Read the model definition and answer for the solid it produces. Units are mm, in the model's axes. Round coordinates to 2 decimals unless told otherwise and drop trailing zeros. Loops run counter-clockwise (first coordinate to the right, second up) from the corner with the lowest first, then second, coordinate; pieces in that order, holes last. Notation, with made-up numbers: (-13.5, 30.5) - (4.5, 30.5) arc R21 cw to (4.5, 45.5) - close; hole circle Ø7 at (62, -37). An arc over 180 degrees is marked (long way). Use CSV: the item, a comma, the result in double quotes. Start each with the question number.
1. Consider line 1 along Y through (x, z) = (0, 1.85); line 2 along Z through (x, y) = (-15, -8.5); line 3 along X through (y, z) = (2, 5.35). Determine where each line is inside the solid, lowest interval first.
2. Find section D-D (x = -11.5). Give the vertices of the cut face in (y, z), and give its area (3 significant figures).
3. Determine the mould class of faces 1 (the cylindrical face through (-0.867, -3.905, 4.479)), 2 (the flat face through (-4.3, 0.3, 3)), 3 (the cylindrical face through (10.2, -0.6, 1.5)) for opening direction X: +X half, -X half, draft (parallel to the pull), parting line (faces both ways), or undercut.
4. Given pin 1 Ø7 at (x, y) = (0, 0) entering from -Z; pin 2 Ø2 at (y, z) = (-9, 2.5) entering from +X; pin 3 Ø2.5 at (x, y) = (0, -11) entering from +Z; pin 4 Ø2 at (y, z) = (-14, 1) entering from +X, each flat-ended and moving along its own axis, determine where each tip first touches the part or whether it passes through.
5. Find section A-A (x = 11). Give the vertices of the cut face in (y, z).
6. Find section B-B (y = 2). Give the vertices of the cut face in (x, z).
7. Find section C-C (z = 4.2). Give the vertices of the cut face in (x, y), and give its area (3 significant figures).
from build123d import *

# Parameters (mm, degrees)
SKETCH1_R           = 18
SKETCH1_R_2         = 1
BOSS_EXTRUDE1_DEPTH = 3
SKETCH2_R           = 4
SKETCH2_R_2         = 3
BOSS_EXTRUDE2_DEPTH = 3
SKETCH3_R           = 3
CUT_EXTRUDE1_DEPTH  = 5


with BuildPart() as part:
    # Sketch1 → Boss-Extrude1 (new body)
    with BuildSketch(Plane.XY):
        Circle(SKETCH1_R)
        with Locations((0, 11)):
            Circle(SKETCH1_R_2, mode=Mode.SUBTRACT)
        with Locations((11, 0)):
            Circle(SKETCH1_R_2, mode=Mode.SUBTRACT)
        with Locations((0, -11)):
            Circle(SKETCH1_R_2, mode=Mode.SUBTRACT)
        with Locations((-11, 0)):
            Circle(SKETCH1_R_2, mode=Mode.SUBTRACT)
    extrude(amount=BOSS_EXTRUDE1_DEPTH)

    # Sketch2 → Boss-Extrude2 (add)
    with BuildSketch(Plane.XY.offset(3)):
        Circle(SKETCH2_R)
        Circle(SKETCH2_R_2, mode=Mode.SUBTRACT)
    extrude(amount=BOSS_EXTRUDE2_DEPTH)

    # Sketch3 → Cut-Extrude1 (cut)
    with BuildSketch(Plane.XY.offset(3)):
        Circle(SKETCH3_R)
    extrude(amount=-CUT_EXTRUDE1_DEPTH, mode=Mode.SUBTRACT)


solid = part.part
Filled sheet:
1,line 1,"y = -18 to -12, -10 to -3, 3 to 10, 12 to 18"
1,line 2,"z = 0 to 3"
1,line 3,"x = -3.46 to -2.24, 2.24 to 3.46"
2,outline,"(-13.85, 0) - (-0.87, 0) - (-0.87, 3) - (-13.85, 3) - close; (0.87, 0) - (13.85, 0) - (13.85, 3) - (0.87, 3) - close"
2,area,"77.9 mm²"
3,face 1,"parting line"
3,face 2,"draft"
3,face 3,"undercut"
4,pin 1,"stops at z = 0"
4,pin 2,"stops at x = 16.12"
4,pin 3,"stops at z = 3"
4,pin 4,"stops at x = 12.45"
5,outline,"(-14.25, 0) - (-1, 0) - (-1, 3) - (-14.25, 3) - close; (1, 0) - (14.25, 0) - (14.25, 3) - (1, 3) - close"
6,outline,"(-17.89, 0) - (-2.24, 0) - (-2.24, 6) - (-3.46, 6) - (-3.46, 3) - (-17.89, 3) - close; (2.24, 0) - (17.89, 0) - (17.89, 3) - (3.46, 3) - (3.46, 6) - (2.24, 6) - close"
7,outline,"circle Ø8 at (0, 0); hole circle Ø6 at (0, 0)"
7,area,"22.0 mm²"
